```python
from build123d import *

# Parameters (mm, degrees)
SKETCH1_W                = 27.6
SKETCH1_H                = 14.4
BOSS_EXTRUDE1_DEPTH      = 1.65
BOSS_EXTRUDE1_DEPTH_BACK = 1.65
FILLET1_R                = 1


with BuildPart() as part:
    # Sketch1 → Boss-Extrude1 (new body, two sides)
    with BuildSketch(Plane(origin=(0, 0, 0), x_dir=(1, 0, 0), z_dir=(0, 1, 0))) as boss_extrude1_sk:
        Rectangle(SKETCH1_W, SKETCH1_H)
    extrude(amount=BOSS_EXTRUDE1_DEPTH)
    extrude(boss_extrude1_sk.sketch, amount=-BOSS_EXTRUDE1_DEPTH_BACK)

    # Fillet1
    fillet1_edges = [part.edges().sort_by_distance(p)[0] for p in [
        (0, 1.65, -7.2),
        (0, -1.65, 7.2),
        (0, 1.65, 7.2),
        (0, -1.65, -7.2),
    ]]
    fillet(fillet1_edges, radius=FILLET1_R)


solid = part.part
```
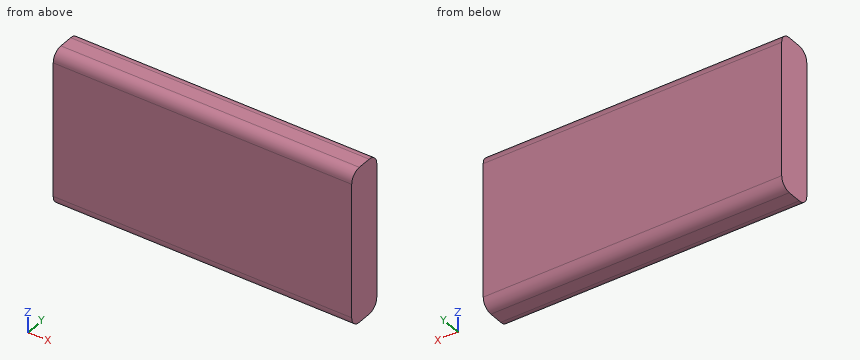
Design review of the part built by this model. Coordinates are the model's own, in mm. Coordinates: 2 decimals unless noted, no trailing zeros. Write each loop counter-clockwise with the first axis right and the second up, starting at its lowest first coordinate (ties: lowest second). Pieces come first, ordered by that corner, then holes. Notation, with made-up numbers: M 1.25,23.5 L 43.25,23.5 A19 cw 43.25,55.5 Z; hole C -33.75,-6 d8. An arc over 180 degrees is marked long. Answer as a JSON object with one key per item and string values.
Item 1: Add section A-A, the plane x = 12.25. Give the boundary of the cut face in (y, z), and give its area (3 significant figures).
Outcome:
{"outline": "M -1.65,-6.2 A1 ccw -0.65,-7.2 L 0.65,-7.2 A1 ccw 1.65,-6.2 L 1.65,6.2 A1 ccw 0.65,7.2 L -0.65,7.2 A1 ccw -1.65,6.2 Z", "area": "46.7 mm²"}
Item 2: Wall thickness on probe 1 along Y at (x, z) = (7, 6.25); probe 2 along Z at (x, y) = (1.75, -1.05); probe 3 along Z at (x, y) = (1.5, -1.5): over which ranges is each line inside the solid? List them lowest first.
Outcome:
{"probe 1": "-1.65 to 1.65", "probe 2": "-7.12 to 7.12", "probe 3": "-6.73 to 6.73"}
Item 3: Add section B-B, the plane y = -1.2. Give the boundary of the cut face in (x, z), and give its area (3 significant figures).
Outcome:
{"outline": "M -13.8,-7.04 L 13.8,-7.04 L 13.8,7.04 L -13.8,7.04 Z", "area": "388 mm²"}
